Read the model definition and answer for the solid it produces. Units are mm, in the model's axes. A direction names the side the tool comes from. Give positions to 0.01 mm unless a question says otherwise; leave off trailing zeros. Loops run counter-clockwise (first coordinate to the right, second up) from the corner with the lowest first, then second, coordinate; pieces in that order, holes last.
(1) Each of these flat-tipped pins is pushed along its axis until it touches: P1, Ø3.5, axis at y = -6, z = 8, coming from the +X side; P2, Ø6, axis at x = 5.5, z = 22, coming from the -Y side; P3, Ø7, axis at x = 11, z = 13, coming from the -Y side; P4, Ø12, axis at x = 17, z = 5, coming from the -Y side. Where does it stop, or does it pass through?
(2) Straight lines are drawn through the part: probe 1 along Z at (x, y) = (12.7, 3.4); probe 2 along Z at (x, y) = (-3.3, -6.35); probe 3 along X at (y, z) = (-2.75, 1.25). For each, find the intervals that lie inside material, in ascending order.
(3) Find section A-A, the plane z = 12.7. State how many separate pieces and enclosed holes the cut face has, then the cut area to 3 significant figures.
(4) Determine the mould class of faces 3 (the face through (16, 3.492, 7)), 4 (the face through (-3.299, -6.557, 14.274)), 5 (the face through (8.7, 3.2, 0)) for opening direction Y: pulls with the +Y half, pulls with the -Y half, needs draft (parallel to the pull), parting line crosses it, or undercut.
(5) Find section C-C, the plane y = -6.35. Write down the section's boundary in (x, z), then the cut area to 3 significant figures.
(6) Which of the six approach directions +Z, -Z, +X, -X, +Y, -Y give full straight-line access (tool end or side, diameter ignored) to faces 1 (the face through (19, 2.858, 10)), 2 (the face through (0.69, -3.1, 12.52))?
(7) Find section D-D, the plane x = 12.7. Write down the section's boundary in (y, z).
```python
from build123d import *

# Parameters (mm, degrees)
F1_DEPTH = 25.4
F3_D     = 3.175
F5_D     = 12.7
F7_D     = 6.35


with BuildPart() as f1:
    # F0 (on Top) → F1 (new body)
    with BuildSketch(Plane.XY):
        with BuildLine():
            ThreePointArc((-3.1115, -1.586229), (0.815672, -3.395914), (3.4925, 0))
            ThreePointArc((3.4925, 0), (3.099247, 1.61004), (2.008046, 2.8575))
            ThreePointArc((2.008046, 2.8575), (1.053028, 3.329968), (0, 3.4925))
            ThreePointArc((0, 3.4925), (-2.46957, 2.46957), (-3.4925, 0))
            ThreePointArc((-3.4925, 0), (-3.395914, -0.815672), (-3.1115, -1.586229))
        make_face()
        with BuildLine():
            ThreePointArc((0, 3.4925), (1.053028, 3.329968), (2.008046, 2.8575))
            Line((2.008046, 2.8575), (25.4, 2.8575))
            Line((25.4, 2.8575), (25.4, 3.4925))
            Line((25.4, 3.4925), (0, 3.4925))
        make_face()
        with BuildLine():
            Line((-3.1115, -12.7), (-3.1115, -1.586229))
            ThreePointArc((-3.1115, -1.586229), (-3.395914, -0.815672), (-3.4925, 0))
            Line((-3.4925, 0), (-3.4925, -12.7))
            Line((-3.4925, -12.7), (-3.1115, -12.7))
        make_face()
    extrude(amount=F1_DEPTH)

    # F3 (through all)
    with Locations(Plane(origin=(-3.4925, 0, 0), x_dir=(0, -1, 0), z_dir=(-1, 0, 0))):
        with Locations((6.35, 12.7)):
            Hole(F3_D / 2)

    # F5 (through all)
    with Locations(Plane(origin=(0, 3.4925, 0), x_dir=(-1, 0, 0), z_dir=(0, 1, 0))):
        with Locations((-12.7, 12.7)):
            Hole(F5_D / 2)

    # F7 (through all)
    with Locations(Plane.XY.offset(25.4)):
        with Locations((0, 0)):
            Hole(F7_D / 2)


solid = f1.part
```
Entries:
1. P1: stops at x = -3.11
1. P2: stops at y = -2.44
1. P3: passes through
1. P4: stops at y = 2.86
2. probe 1: z = 0 to 6.35, 19.05 to 25.4
2. probe 2: z = 0 to 11.11, 14.29 to 25.4
2. probe 3: x = -3.49 to -3.11, -2.15 to -1.59, 1.59 to 2.15
3. separate pieces: 3
3. enclosed holes: 1
3. area: 17.1 mm2
4. face 3: pulls with the +Y half
4. face 4: undercut
4. face 5: needs draft
5. outline: (-3.49, 0) - (-3.11, 0) - (-3.11, 11.11) - (-3.49, 11.11) - close; (-3.49, 14.29) - (-3.11, 14.29) - (-3.11, 25.4) - (-3.49, 25.4) - close
5. area: 8.47 mm2
6. face 1: +Z, -Z, +X
6. face 2: +Z, -Z
7. outline: (2.86, 0) - (3.49, 0) - (3.49, 6.35) - (2.86, 6.35) - close; (2.86, 19.05) - (3.49, 19.05) - (3.49, 25.4) - (2.86, 25.4) - close
